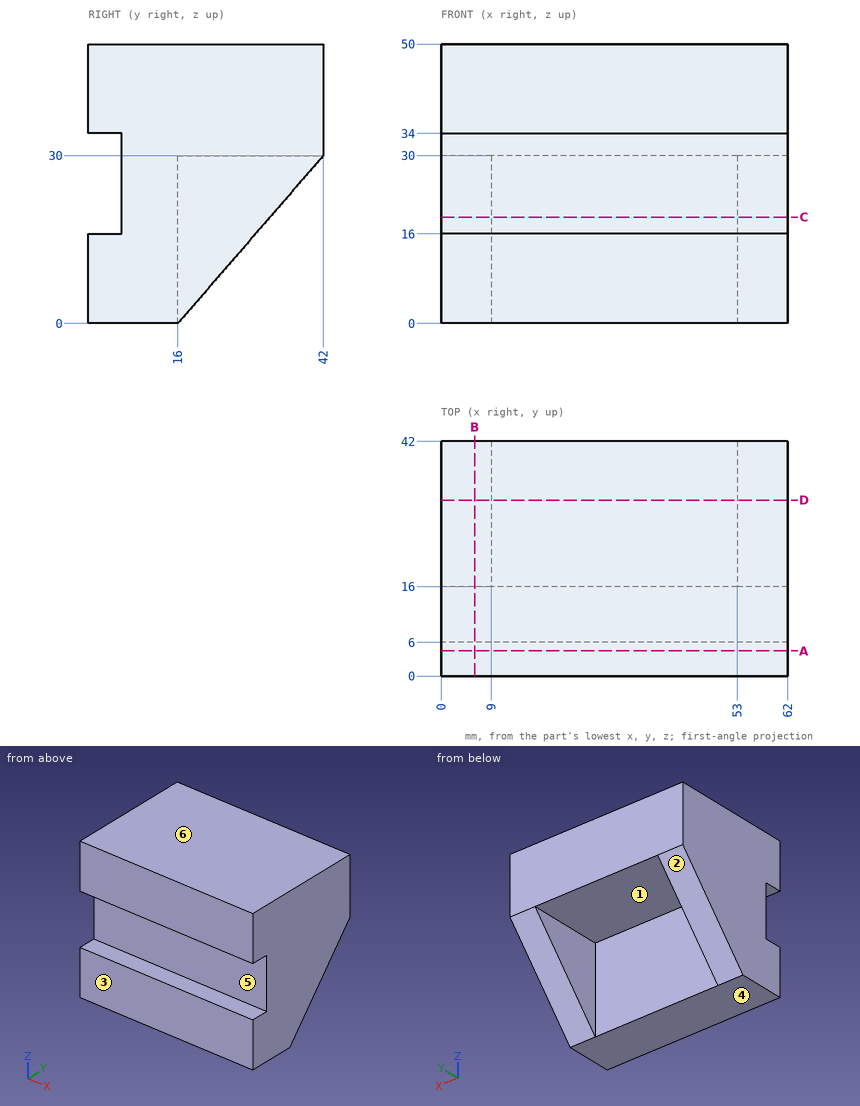
The figure shows three views and two pictorial views of one solid part (mm, origin at its lowest corner). Answer the questions. A direction names the side the tool comes from. Coordinates: 2 decimals unless noted, no trailing zeros. Loops run counter-clockwise (first coordinate to the right, second up) from the corner with the lowest first, then second, coordinate; pieces in that order, holes last.
(1) The mould has two halves that part along Z. Classify the marked faces 3, 4, 5 and 6: released by +Z, released by -Z, zero draft, split by the parting line, or undercut.
Solution:
face 3: zero draft
face 4: released by -Z
face 5: undercut
face 6: released by +Z
(2) The part is cut by section A-A (y = 4.5). Determine the outline of the cut face in (x, z).
Solution:
outline: (0, 0) - (62, 0) - (62, 16) - (0, 16) - close; (0, 34) - (62, 34) - (62, 50) - (0, 50) - close
(3) The part is cut by section D-D (y = 31.5). Determine the outline of the cut face in (x, z).
Solution:
outline: (0, 17.88) - (9, 17.88) - (9, 30) - (53, 30) - (53, 17.88) - (62, 17.88) - (62, 50) - (0, 50) - close
(4) The part is cut by section B-B (x = 6). Determine the outline of the cut face in (y, z).
Solution:
outline: (0, 0) - (16, 0) - (42, 30) - (42, 50) - (0, 50) - (0, 34) - (6, 34) - (6, 16) - (0, 16) - close
(5) Consider line 1 along Z through (x, y) = (25, 5); line 2 along X through (y, z) = (26, 24); line 3 along Z through (x, y) = (16.5, 19). Determine where each line is inside the solid, lowest interval first.
Solution:
line 1: z = 0 to 16, 34 to 50
line 2: x = 0 to 9, 53 to 62
line 3: z = 30 to 50
(6) A tool of negligible diameter and unlimited length cuts with its end or side. For the marked faces 1 and 2, from which of +Z, -Z, +X, -X, +Y, -Y can it reach the whole face along a straight path? Write none if from no direction.
Solution:
face 1: -Z, +Y
face 2: -Z, +X, -X, +Y
(7) Flat-ended cylindrical pins translate along their axes: pin 1 Ø2 at (x, z) = (18, 24) entering from +Y; pin 2 Ø12 at (x, y) = (46.5, 25) entering from -Z; pin 3 Ø8 at (y, z) = (30.5, 9.5) entering from -X. Find the tip coordinate at first contact, or state that the pin passes through.
Solution:
pin 1: stops at y = 16
pin 2: stops at z = 30
pin 3: passes through
(8) The part is cut by section C-C (z = 19). Determine the outline of the cut face in (x, y), and give its area (3 significant figures).
Solution:
outline: (0, 6) - (62, 6) - (62, 32.47) - (53, 32.47) - (53, 16) - (9, 16) - (9, 32.47) - (0, 32.47) - close
area: 916 mm2
